Geometry check sheet. Reference: drawing and pictorial views, mm from the part's lowest x, y, z. Give positions to 0.01 mm unless a question says otherwise; leave off trailing zeros. Order: outer loops, then holes, each group sorted by start corner. A loop starts at its lowest first (then second) coordinate and runs counter-clockwise, first axis right, second up.
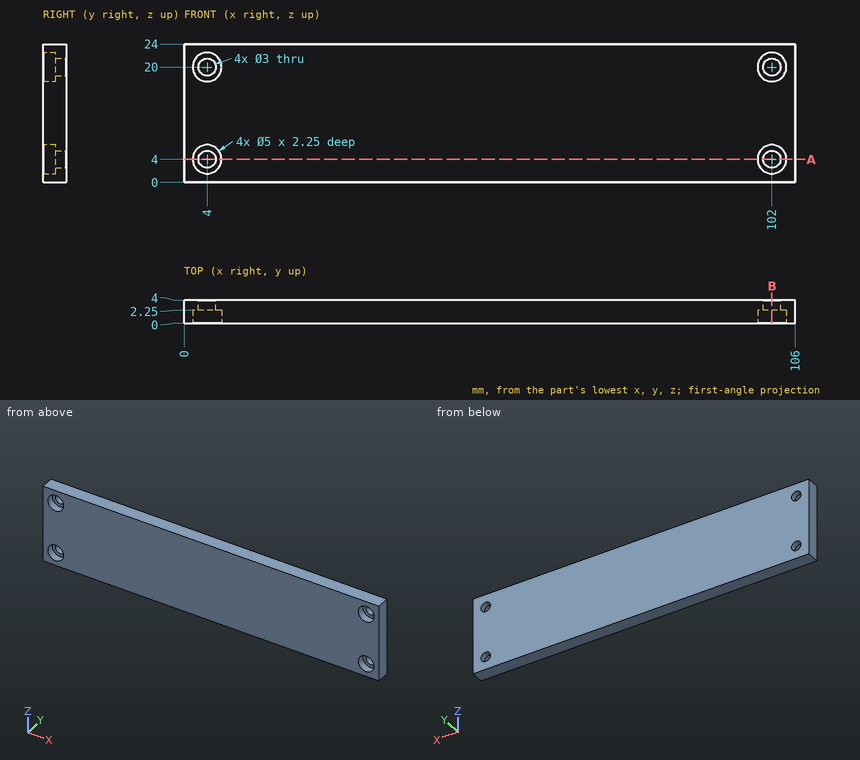
(1) Cross-section at A-A on z = 4. Enter the section's corners in (x, y).
Response values:
outline: (0, 0) - (1.5, 0) - (1.5, 2.25) - (2.5, 2.25) - (2.5, 4) - (0, 4) - close; (5.5, 2.25) - (6.5, 2.25) - (6.5, 0) - (99.5, 0) - (99.5, 2.25) - (100.5, 2.25) - (100.5, 4) - (5.5, 4) - close; (103.5, 2.25) - (104.5, 2.25) - (104.5, 0) - (106, 0) - (106, 4) - (103.5, 4) - close
(2) Gauge pin test, flat end, axial feed: pin 1 Ø4 at (x, z) = (4, 20) entering from -Y. Record the tip position at first contact, or that the pin passes through.
Response values:
pin 1: stops at y = 2.25
(3) Cross-section at B-B on x = 102. Enter the section's corners in (y, z), then the cut area to 3 significant figures.
Response values:
outline: (0, 0) - (4, 0) - (4, 2.5) - (2.25, 2.5) - (2.25, 1.5) - (0, 1.5) - close; (0, 6.5) - (2.25, 6.5) - (2.25, 5.5) - (4, 5.5) - (4, 18.5) - (2.25, 18.5) - (2.25, 17.5) - (0, 17.5) - close; (0, 22.5) - (2.25, 22.5) - (2.25, 21.5) - (4, 21.5) - (4, 24) - (0, 24) - close
area: 63.0 mm2
(4) Material ranges on L1, parallel to Z at x = 102, y = 0.8; L2, parallel to Z at x = 102, y = 3.3; L3, parallel to X at y = 2.75, z = 4, recorded low to high.
Response values:
L1: z = 0 to 1.5, 6.5 to 17.5, 22.5 to 24
L2: z = 0 to 2.5, 5.5 to 18.5, 21.5 to 24
L3: x = 0 to 2.5, 5.5 to 100.5, 103.5 to 106
